Here's how the part is built. I have some questions about the finished solid (model axes, mm). Give positions to 0.01 mm unless a question says otherwise; leave off trailing zeros. Write each loop counter-clockwise with the first axis right and the second up, starting at its lowest first coordinate (ties: lowest second). Pieces come first, ordered by that corner, then holes. Notation, with made-up numbers: (17, 23.25) -> (38, 23.25) arc R24 cw to (38, 46.25) -> close; hole circle Ø5 at (46, 35.25). An arc over 180 degrees is marked (long way). Return JSON: item names as keys, results as strings.
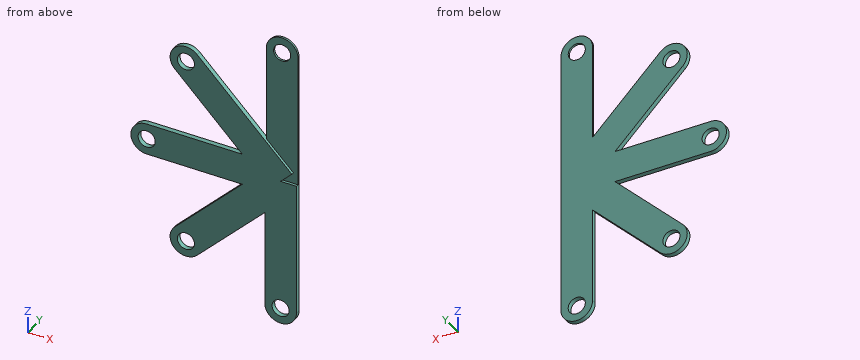
Autodesk Inventor part; units mm, degrees
ref_plane "to_body_XY" through (0, 0, 0) normal (0, -1, 0) x (1, 0, 0)
ref_plane "to_body_YZ" through (0, 0, 0) normal (1, 0, 0) x (0, 0, 1)
ref_plane "to_body_ZX" through (0, 0, 0) normal (0, 0, 1) x (0, -1, 0)
sketch "Sketch_1" plane through (0, 0, 0) normal (0, 1, 0) x (-1, 0, 0)
  arc A0 (2.4003, 20.2946) -> (-2.4003, 20.2946) centre (0, 20.2946) ccw
  line L0 (-2.4003, 20.2946) -> (-2.4003, 0)
  line L1 (-2.4003, 0) -> (2.4003, 0)
  line L2 (2.4003, 0) -> (2.4003, 20.2946)
  circle A1 centre (0, 20.2946) radius 1.2954
extrude "Extrusion1" add sketch "Sketch_1" against normal blind 0.3048
sketch "Sketch_2" plane through (0, 0, 0) normal (0, 1, 0) x (-1, 0, 0)
  arc A0 (16.0477, 12.6532) -> (12.6532, 16.0477) centre (14.3504, 14.3504) ccw
  line L0 (12.6532, 16.0477) -> (-1.6973, 1.6973)
  line L1 (-1.6973, 1.6973) -> (1.6973, -1.6973)
  line L2 (1.6973, -1.6973) -> (16.0477, 12.6532)
  circle A1 centre (14.3504, 14.3504) radius 1.2954
extrude "Extrusion2" add sketch "Sketch_2" against normal blind 0.7112
sketch "Sketch_3" plane through (0, 0, 0) normal (0, 1, 0) x (-1, 0, 0)
  arc A0 (20.2946, -2.4003) -> (20.2946, 2.4003) centre (20.2946, 0) ccw
  line L0 (20.2946, 2.4003) -> (0, 2.4003)
  line L1 (0, 2.4003) -> (0, -2.4003)
  line L2 (0, -2.4003) -> (20.2946, -2.4003)
  circle A1 centre (20.2946, 0) radius 1.2954
extrude "Extrusion3" add sketch "Sketch_3" against normal blind 0.7112
sketch "Sketch_4" plane through (0, 0, 0) normal (0, 1, 0) x (-1, 0, 0)
  arc A0 (12.6532, -16.0477) -> (16.0477, -12.6532) centre (14.3504, -14.3504) ccw
  line L0 (16.0477, -12.6532) -> (1.6973, 1.6973)
  line L1 (1.6973, 1.6973) -> (-1.6973, -1.6973)
  line L2 (-1.6973, -1.6973) -> (12.6532, -16.0477)
  circle A1 centre (14.3504, -14.3504) radius 1.2954
extrude "Extrusion4" add sketch "Sketch_4" against normal blind 0.7112
sketch "Sketch_5" plane through (0, 0, 0) normal (0, 1, 0) x (-1, 0, 0)
  line L0 (2.4003, -20.2946) -> (2.4003, 0)
  line L1 (2.4003, 0) -> (-2.4003, 0)
  line L2 (-2.4003, 0) -> (-2.4003, -20.2946)
  arc A0 (-2.4003, -20.2946) -> (2.4003, -20.2946) centre (0, -20.2946) ccw
  circle A1 centre (0, -20.2946) radius 1.2954
extrude "Extrusion5" add sketch "Sketch_5" against normal blind 0.7112
ref_plane "to_body_XY" through (0, 0, 0) normal (0, -1, 0) x (1, 0, 0)
ref_plane "to_body_YZ" through (0, 0, 0) normal (1, 0, 0) x (0, 0, 1)
ref_plane "to_body_ZX" through (0, 0, 0) normal (0, 0, 1) x (0, -1, 0)
properties part number "HS13Z-trmnls"
1. Suppose I cut it at C-C, the plane x = -3. List the corners of the cut face in (y, z) for me, and give its area (3 significant figures).
Taken from the geometry:
{"outline": "(-0.71, -6.39) -> (0, -6.39) -> (0, 6.39) -> (-0.71, 6.39) -> close", "area": "9.10 mm²"}
2. For pin 1 Ø1 at (x, z) = (-15.5, 9) entering from -Y; pin 2 Ø4 at (x, z) = (1, 11.5) entering from -Y, each with a flat end and sliding along its axis, tell me the tip position at first contact or that it passes through.
Taken from the geometry:
{"pin 1": "passes through", "pin 2": "stops at y = -0.3"}
3. If I drill on line 1 (Z direction, x = -15.75, y = -0.6); line 2 (Z direction, x = -13, y = -0.65); line 3 (Z direction, x = -15.5, y = -0.6), over which ranges is the centre line in solid material (lowest first)? Write a range as [from, to].
Taken from the geometry:
{"line 1": "z = [-16.3, -12.36], [-2.4, 2.4], [12.36, 16.3]", "line 2": "z = [-16.33, -9.61], [-2.4, 2.4], [9.61, 16.33]", "line 3": "z = [-16.46, -14.95], [-13.75, -12.11], [-2.4, 2.4], [12.11, 13.75], [14.95, 16.46]"}
4. Suppose I cut it at B-B, the plane y = -0.6. List the corners of the cut face in (x, z) for me, and give its area (3 significant figures).
Taken from the geometry:
{"outline": "(-20.29, -2.4) -> (-5.79, -2.4) -> (-16.05, -12.65) arc R2.4 ccw to (-12.65, -16.05) -> (-2.4, -5.79) -> (-2.4, -20.29) arc R2.4 ccw to (2.4, -20.29) -> (2.4, 0) -> (0, 0) -> (1.7, 1.7) -> (-12.65, 16.05) arc R2.4 ccw to (-16.05, 12.65) -> (-5.79, 2.4) -> (-20.29, 2.4) arc R2.4 ccw to start; hole circle Ø2.59 at (-20.29, 0); hole circle Ø2.59 at (-14.35, -14.35); hole circle Ø2.59 at (-14.35, 14.35); hole circle Ø2.59 at (0, -20.29)", "area": "363 mm²"}
5. Suppose I cut it at A-A, the plane x = -8.25. List the corners of the cut face in (y, z) for me.
Taken from the geometry:
{"outline": "(-0.71, -11.64) -> (0, -11.64) -> (0, -4.86) -> (-0.71, -4.86) -> close; (-0.71, -2.4) -> (0, -2.4) -> (0, 2.4) -> (-0.71, 2.4) -> close; (-0.71, 4.86) -> (0, 4.86) -> (0, 11.64) -> (-0.71, 11.64) -> close"}
